```python
from build123d import *

# Parameters (mm, degrees)
ESBO_O1_W                = 34.2
ESBO_O1_H                = 25.4
RESSALTO_EXTRUS_O1_DEPTH = 0.45
ESBO_O2_R                = 0.5
CORTE_EXTRUS_O1_DEPTH    = 22.319240137
FILETE1_R                = 1


with BuildPart() as part:
    # Esboço1 → Ressalto-extrusão1 (new, symmetric)
    with BuildSketch(Plane(origin=(0, 0, 0), x_dir=(1, 0, 0), z_dir=(0, 1, 0))):
        Rectangle(ESBO_O1_W, ESBO_O1_H)
    extrude(amount=RESSALTO_EXTRUS_O1_DEPTH, both=True)

    # Esboço2 → Corte-extrusão1 (cut, through all)
    with BuildSketch(Plane(origin=(0, 0.45, 0), x_dir=(1, 0, 0), z_dir=(0, 1, 0))):
        with Locations(Location((15.1, 1.27, 0), (0, 0, 270))):
            Circle(ESBO_O2_R)
        with Locations(Location((15.1, -1.27, 0), (0, 0, 270))):
            Circle(ESBO_O2_R)
        with Locations(Location((-2.98, 10.7, 0), (0, 0, 270))):
            Circle(ESBO_O2_R)
        with Locations(Location((-0.44, 10.7, 0), (0, 0, 270))):
            Circle(ESBO_O2_R)
        with Locations(Location((3.56, 10.7, 0), (0, 0, 270))):
            Circle(ESBO_O2_R)
        with Locations(Location((6.1, 10.7, 0), (0, 0, 270))):
            Circle(ESBO_O2_R)
        with Locations(Location((-15.1, 2.62, 0), (0, 0, 270))):
            Circle(ESBO_O2_R)
        with Locations(Location((-15.1, 5.16, 0), (0, 0, 270))):
            Circle(ESBO_O2_R)
        with Locations(Location((-15.1, 8.16, 0), (0, 0, 270))):
            Circle(ESBO_O2_R)
        with Locations(Location((-15.1, 10.7, 0), (0, 0, 270))):
            Circle(ESBO_O2_R)
        with Locations(Location((6.1, -10.7, 0), (0, 0, 90))):
            Circle(ESBO_O2_R)
        with Locations(Location((3.56, -10.7, 0), (0, 0, 90))):
            Circle(ESBO_O2_R)
        with Locations(Location((-0.44, -10.7, 0), (0, 0, 90))):
            Circle(ESBO_O2_R)
        with Locations(Location((-2.98, -10.7, 0), (0, 0, 90))):
            Circle(ESBO_O2_R)
        with Locations(Location((-15.1, -10.7, 0), (0, 0, 90))):
            Circle(ESBO_O2_R)
        with Locations(Location((-15.1, -8.16, 0), (0, 0, 90))):
            Circle(ESBO_O2_R)
        with Locations(Location((-15.1, -5.16, 0), (0, 0, 90))):
            Circle(ESBO_O2_R)
        with Locations(Location((-15.1, -2.62, 0), (0, 0, 90))):
            Circle(ESBO_O2_R)
    extrude(amount=-CORTE_EXTRUS_O1_DEPTH, mode=Mode.SUBTRACT)

    # Filete1
    filete1_edges = [part.edges().sort_by_distance(p)[0] for p in [
        (-17.1, 0, -12.7),
        (17.1, 0, -12.7),
        (17.1, 0, 12.7),
        (-17.1, 0, 12.7),
    ]]
    fillet(filete1_edges, radius=FILETE1_R)


solid = part.part
```
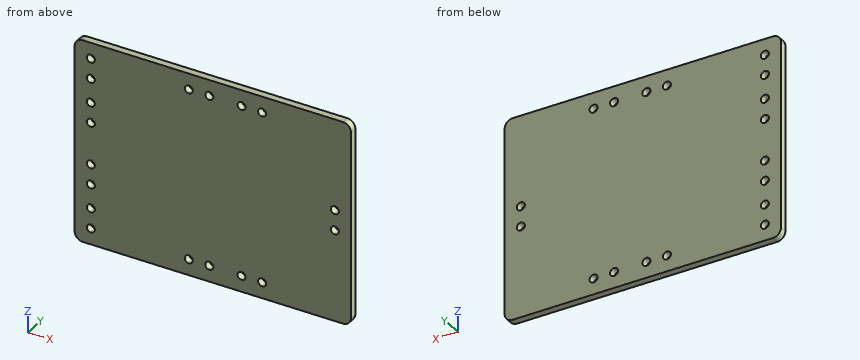
Geometry check sheet. Reference: the model listing, model coordinates, mm. Round coordinates to 2 decimals unless told otherwise and drop trailing zeros. Write each loop counter-clockwise with the first axis right and the second up, starting at its lowest first coordinate (ties: lowest second). Pieces come first, ordered by that corner, then holes. Notation, with made-up numbers: (-8.75, -36.5) -> (41.25, -36.5) arc R21 cw to (41.25, -32.5) -> close; hole circle Ø11 at (82, 16.5). An arc over 180 degrees is marked (long way). Put each result on its own line as item: value.
1) Cross-section at B-B, the plane z = -1.27. Enter the section's corners in (x, y), plus the area to 3 significant figures.
Recorded:
outline: (-17.1, -0.45) -> (14.6, -0.45) -> (14.6, 0.45) -> (-17.1, 0.45) -> close; (15.6, -0.45) -> (17.1, -0.45) -> (17.1, 0.45) -> (15.6, 0.45) -> close
area: 29.9 mm2
2) Thickness scan on probe 1 along X at (y, z) = (-0.1, -10.7); probe 2 along Z at (x, y) = (6, -0.1); probe 3 along X at (y, z) = (0.1, -7.75). Record the ranges inside material, lowest first. Write a range as from..to.
Recorded:
probe 1: x = -17.1..-15.6, -14.6..-3.48, -2.48..-0.94, 0.06..3.06, 4.06..5.6, 6.6..17.1
probe 2: z = -12.7..-11.19, -10.21..10.21, 11.19..12.7
probe 3: x = -17.1..-15.39, -14.81..17.1
3) Cross-section at A-A, the plane x = 6.1. Enter the section's corners in (y, z), plus the area to 3 significant figures.
Recorded:
outline: (-0.45, -12.7) -> (0.45, -12.7) -> (0.45, -11.2) -> (-0.45, -11.2) -> close; (-0.45, -10.2) -> (0.45, -10.2) -> (0.45, 10.2) -> (-0.45, 10.2) -> close; (-0.45, 11.2) -> (0.45, 11.2) -> (0.45, 12.7) -> (-0.45, 12.7) -> close
area: 21.1 mm2
4) Cross-section at C-C, the plane y = 0.05. Give the number of separate pieces and of enclosed holes in the cut face, plus the area to 3 significant figures.
Recorded:
separate pieces: 1
enclosed holes: 18
area: 854 mm2
